from build123d import *

# Parameters (mm, degrees)
SKETCH_1_W          = 60
SKETCH_1_H          = 40
EXTRUDE_1_DEPTH     = 20
SKETCH_2_R          = 7.5
EXTRUDE_2_DEPTH     = 15
SKETCH_3_W          = 15
SKETCH_3_H          = 5
CUT_EXTRUDE_1_DEPTH = 42.231056256
SKETCH_4_W          = 10
SKETCH_4_H          = 15
CUT_EXTRUDE_2_DEPTH = 73.284161474
CHAMFER_1_SIZE      = 5


with BuildPart() as part:
    # Эскиз1 → Бобышка-Вытянуть1 (new body)
    with BuildSketch(Plane.XY):
        Rectangle(SKETCH_1_W, SKETCH_1_H)
    extrude(amount=EXTRUDE_1_DEPTH)

    # Эскиз2 → Бобышка-Вытянуть2 (add)
    with BuildSketch(Plane.XY.offset(20)):
        with Locations(Location((0, 0, 0), (0, 0, 180))):
            Circle(SKETCH_2_R)
    extrude(amount=EXTRUDE_2_DEPTH)

    # Эскиз3 → Вырез-Вытянуть1 (cut, through all)
    with BuildSketch(Plane.XY.offset(20)):
        with Locations((0, -17.5)):
            Rectangle(SKETCH_3_W, SKETCH_3_H)
    cut_extrude_1 = extrude(amount=-CUT_EXTRUDE_1_DEPTH, mode=Mode.SUBTRACT)

    # Зеркальное отражение1: Вырез-Вытянуть1 across plane
    add(cut_extrude_1.mirror(Plane.ZX), mode=Mode.SUBTRACT)

    # Эскиз4 → Вырез-Вытянуть2 (cut, through all)
    with BuildSketch(Plane.ZY.offset(30)):
        with Locations((5, 0)):
            Rectangle(SKETCH_4_W, SKETCH_4_H)
    extrude(amount=-CUT_EXTRUDE_2_DEPTH, mode=Mode.SUBTRACT)

    # Фаска1
    chamfer_1_edges = [part.edges().sort_by_distance(p)[0] for p in [
        (30, -20, 10),
        (-30, -20, 10),
        (-30, 20, 10),
        (30, 20, 10),
    ]]
    chamfer(chamfer_1_edges, length=CHAMFER_1_SIZE)


solid = part.part
Input: part model. Units: mm. Frame: model coordinates. A direction names the side the tool comes from. Give positions to 0.01 mm unless a question says otherwise; leave off trailing zeros. Write each loop counter-clockwise with the first axis right and the second up, starting at its lowest first coordinate (ties: lowest second). Pieces come first, ordered by that corner, then holes. Notation, with made-up numbers: M 50.25,46.25 L 56.25,46.25 A21 ccw 56.25,55.25 Z; hole C 68,2 d2. An arc over 180 degrees is marked long. Write item = value, one per line. Start each with the question number.
1) Cut plane C-C on y = 0. Return the cut outline in (x, z), then the cut area to 3 significant figures.
2) Reachability of faces 5 (the flat face through (0, 0, 10)), 6 (the flat face through (0, -15, 10)), 7 (the flat face through (0, 15, 10)), 8 (the flat face through (30, 0, 12)), 9 (the flat face through (-30, 0, 12)) from +Z, -Z, +X, -X, +Y, -Y: full face, straight path, thin tool, end or side. Return the list, or none.
3) First-contact query: pin 1 Ø4 at (x, z) = (-4, 20.5) entering from -Y; pin 2 Ø1.5 at (x, y) = (-1.5, -4.5) entering from -Z; pin 3 Ø4 at (y, z) = (18, 11) entering from -X; pin 4 Ø4 at (y, z) = (15.5, 15.5) entering from +X. Flat tips, straight axial feed; report the tip coordinate or a pass-through.
4) Cut plane D-D on x = 0. Return the cut outline in (y, z), then the cut area to 3 significant figures.
5) Cut plane A-A on z = 15.5. Return the cut outline in (x, y), then the cut area to 3 significant figures.
6) Material intervals for line 1 along Y through (x, z) = (18.5, 7); line 2 along Y through (x, z) = (1, 3); line 3 along Z through (x, y) = (-6.5, 13.5), sorted ascending. Write a range as [from, to].
7) Draft query along Y for faces 1 (the flat face through (-27, -18, 10)), 2 (the flat face through (0, -7.5, 5)), 3 (the flat face through (-27, 18, 10)), 4 (the flat face through (7.5, 18, 10)). Return one class per face: +Y half, -Y half, draft (parallel to the pull), parting line (faces both ways), or undercut.
8) Cut plane B-B on x = 22. Return the cut outline in (y, z).
Solved:
q1.outline = M -30,10 L 30,10 L 30,20 L 7.5,20 L 7.5,35 L -7.5,35 L -7.5,20 L -30,20 Z
q1.area = 825 mm2
q2.face_5 = -Z, +X, -X
q2.face_6 = +Z, -Z, -Y
q2.face_7 = +Z, -Z, +Y
q2.face_8 = +Z, -Z, +X, +Y, -Y
q2.face_9 = +Z, -Z, -X, +Y, -Y
q3.pin_1 = -15
q3.pin_2 = 10
q3.pin_3 = -29
q3.pin_4 = 30
q4.outline = M -15,0 L -7.5,0 L -7.5,10 L 7.5,10 L 7.5,0 L 15,0 L 15,20 L 7.5,20 L 7.5,35 L -7.5,35 L -7.5,20 L -15,20 Z
q4.area = 675 mm2
q5.outline = M -30,-15 L -25,-20 L -7.5,-20 L -7.5,-15 L 7.5,-15 L 7.5,-20 L 25,-20 L 30,-15 L 30,15 L 25,20 L 7.5,20 L 7.5,15 L -7.5,15 L -7.5,20 L -25,20 L -30,15 Z
q5.area = 2,200 mm2
q6.line_1 = [-20, -7.5], [7.5, 20]
q6.line_2 = [-15, -7.5], [7.5, 15]
q6.line_3 = [0, 20]
q7.face_1 = -Y half
q7.face_2 = undercut
q7.face_3 = +Y half
q7.face_4 = draft
q8.outline = M -20,0 L -7.5,0 L -7.5,10 L 7.5,10 L 7.5,0 L 20,0 L 20,20 L -20,20 Z
